from build123d import *

# Parameters (mm, degrees)
SKETCH1_W           = 57.15
SKETCH1_H           = 38.1
SKETCH1_W_2         = 40.64
SKETCH1_H_2         = 26.035
BOSS_EXTRUDE1_DEPTH = 16.66875
CUT_EXTRUDE1_DEPTH  = 30.95625
SKETCH5_W           = 19.05
SKETCH5_H           = 11.1125
CUT_EXTRUDE2_DEPTH  = 57.15
SKETCH6_R           = 2.1828125
CUT_EXTRUDE3_DEPTH  = 19.05
SKETCH9_W           = 57.15
SKETCH9_H           = 28.575
BOSS_EXTRUDE2_DEPTH = 22.225
SKETCH10_R          = 1.5875
CUT_EXTRUDE4_DEPTH  = 28.575
CUT_EXTRUDE6_REACH  = 46.45
SKETCH12_W          = 44.45
SKETCH12_H          = 19.05
FILLET1_R           = 3.175


with BuildPart() as part:
    # Sketch1 → Boss-Extrude1 (new body, symmetric)
    with BuildSketch(Plane.XY):
        Rectangle(SKETCH1_W, SKETCH1_H)
        Rectangle(SKETCH1_W_2, SKETCH1_H_2, mode=Mode.SUBTRACT)
    extrude(amount=BOSS_EXTRUDE1_DEPTH, both=True)

    # Sketch3 → Cut-Extrude1 (cut)
    with BuildSketch(Plane(origin=(0, 19.05, 0), x_dir=(1, 0, 0), z_dir=(0, 1, 0))):
        with BuildLine():
            Line((20.32, -10.16), (20.32, 9.36625))
            ThreePointArc((20.32, 9.36625), (20.087516008, 9.927516008), (19.52625, 10.16))
            Line((19.52625, 10.16), (-19.52625, 10.16))
            ThreePointArc((-19.52625, 10.16), (-20.087516008, 9.927516008), (-20.32, 9.36625))
            Line((-20.32, 9.36625), (-20.32, -10.16))
            Line((-20.32, -10.16), (-20.32, -16.66875))
            Line((-20.32, -16.66875), (20.32, -16.66875))
            Line((20.32, -16.66875), (20.32, -10.16))
        make_face()
    extrude(amount=-CUT_EXTRUDE1_DEPTH, mode=Mode.SUBTRACT)

    # Sketch5 → Cut-Extrude2 (cut)
    with BuildSketch(Plane.ZY.offset(28.575)):
        with Locations((0, -7.46125)):
            Rectangle(SKETCH5_W, SKETCH5_H)
    extrude(amount=-CUT_EXTRUDE2_DEPTH, mode=Mode.SUBTRACT)

    # Sketch6 → Cut-Extrude3 (cut)
    with BuildSketch(Plane(origin=(0, 19.05, 0), x_dir=(1, 0, 0), z_dir=(0, 1, 0))):
        with Locations((-24.0109375, -4.7625)):
            Circle(SKETCH6_R)
        with Locations((-24.0109375, 4.7625)):
            Circle(SKETCH6_R)
        with Locations((24.209375, -4.7625)):
            Circle(SKETCH6_R)
        with Locations((24.209375, 4.7625)):
            Circle(SKETCH6_R)
    extrude(amount=-CUT_EXTRUDE3_DEPTH, mode=Mode.SUBTRACT)

    # Sketch9 → Boss-Extrude2 (add, symmetric)
    with BuildSketch(Plane.XY):
        with Locations((0, -27.305)):
            Rectangle(SKETCH9_W, SKETCH9_H)
    extrude(amount=BOSS_EXTRUDE2_DEPTH, both=True)

    # Sketch10 → Cut-Extrude4 (cut)
    with BuildSketch(Plane(origin=(0, -13.0175, 0), x_dir=(1, 0, 0), z_dir=(0, 1, 0))):
        with Locations((-25.4, 19.05)):
            Circle(SKETCH10_R)
        with Locations((25.4, 19.05)):
            Circle(SKETCH10_R)
        with Locations((-25.4, -19.05)):
            Circle(SKETCH10_R)
        with Locations((25.4, -19.05)):
            Circle(SKETCH10_R)
    extrude(amount=-CUT_EXTRUDE4_DEPTH, mode=Mode.SUBTRACT)

    # Sketch12 → Cut-Extrude6 (cut, up to next)
    with BuildSketch(Plane.XY.offset(22.225), mode=Mode.PRIVATE) as cut_extrude6_sk1:
        with Locations((0, -27.305)):
            Rectangle(SKETCH12_W, SKETCH12_H)
    cut_extrude6_tool1 = extrude(cut_extrude6_sk1.sketch, amount=-CUT_EXTRUDE6_REACH, mode=Mode.PRIVATE) & part.part
    add(cut_extrude6_tool1.solids().sort_by_distance((0, -27.305, 22.225))[0], mode=Mode.SUBTRACT)

    # Fillet1
    fillet1_edges = [part.edges().sort_by_distance(p)[0] for p in [
        (28.575, 3.01625, -16.66875),
        (28.575, 3.01625, 16.66875),
        (-28.575, -27.305, -22.225),
        (28.575, -27.305, -22.225),
        (-28.575, -27.305, 22.225),
        (28.575, -27.305, 22.225),
        (20.32, 0, -16.66875),
        (-22.225, -36.83, 0),
        (-22.225, -17.78, 0),
        (22.225, -17.78, 0),
        (22.225, -36.83, 0),
        (-20.32, 0, -16.66875),
        (20.32, 3.01625, 16.66875),
        (-20.32, 3.01625, 16.66875),
        (-28.575, 3.01625, 16.66875),
        (-28.575, 3.01625, -16.66875),
        (24.4475, -13.0175, 9.525),
        (24.4475, -1.905, -9.525),
        (24.4475, -1.905, 9.525),
        (24.4475, -13.0175, -9.525),
        (-24.4475, -1.905, 9.525),
        (-24.4475, -13.0175, 9.525),
        (-24.4475, -13.0175, -9.525),
        (-24.4475, -1.905, -9.525),
    ]]
    fillet(fillet1_edges, radius=FILLET1_R)


solid = part.part
Could you check a few things on this model? Use its own coordinates, in mm. A direction names the side the tool comes from. Coordinates: 2 decimals unless noted, no trailing zeros.
Q1. Suppose I cut it at A-A on y = -24. Give the number of separate pieces and of enclosed holes in the cut face, and give its area (3 significant figures).
Q2. Which directions (+Z, -Z, +X, -X, +Y, -Y) give clear straight access to the entire face, cutting with the end or side of a thin tool? Please do faces 5 (the cylindrical face through (-27.67, 3.241, 15.714)), 6 (the cylindrical face through (-21.93, 9.66, 4.11)), 7 (the cylindrical face through (27.67, 3.241, 15.714)).
Q3. Thinking about a two-plate mould opening in Y: for faces 1 (the flat face through (24, -1.905, 0)), 2 (the flat face through (2, 19.05, -11)), 3 (the cylindrical face through (27.62, 3.241, -15.763)), 4 (the cylindrical face through (21.27, -35.925, -0.311)), which applies, released by +Y, released by -Y, zero draft, split by the parting line, or undercut?
Q4. Please list where these lines run through material, in increasing order: L1, parallel to Z at x = 25.4, y = -25.75 (1 decimal); L2, parallel to X at y = -30, z = 19 (3 decimals); L3, parallel to Y at x = 9, z = -9.5.
Q5. Will these pins go through, and if not, where does the flat tip stop? pin 1 (5 mm diameter, centred on x = 25.5, y = -7, fed in from +Z); pin 2 (2 mm diameter, centred on x = 23.5, z = 4, fed in from +Y); pin 3 (5 mm diameter, centred on x = 23, y = -8, fed in from -Z).
Answer:
1. separate pieces: 2
1. enclosed holes: 4
1. area: 524 mm2
2. face 5: +Z, -X, +Y
2. face 6: +Y
2. face 7: +Z, +X, +Y
3. face 1: undercut
3. face 2: released by +Y
3. face 3: zero draft
3. face 4: undercut
4. L1: z = -22.2 to -20.6, -17.5 to 17.5, 20.6 to 22.2
4. L2: x = -28.575 to -26.987, -23.813 to -22.225, 22.225 to 23.813, 26.987 to 28.575
4. L3: y = -41.59 to -36.83, -17.78 to -13.02
5. pin 1: stops at z = 16.67
5. pin 2: stops at y = 0
5. pin 3: stops at z = -16.67
